Build history of the part. All positions in model axes, mm. Face numbers are marked on the shaded views. A direction names the side the tool comes from. Round coordinates to 2 decimals unless told otherwise and drop trailing zeros. Loops run counter-clockwise (first coordinate to the right, second up) from the corner with the lowest first, then second, coordinate; pieces in that order, holes last. Notation, with made-up numbers: (-35.75, 60.25) - (18.25, 60.25) arc R27 ccw to (18.25, 93.25) - close; hole circle Ø7 at (34, 83.5). An arc over 180 degrees is marked (long way). Put each result on its own line as item: value. Start each with the question number.
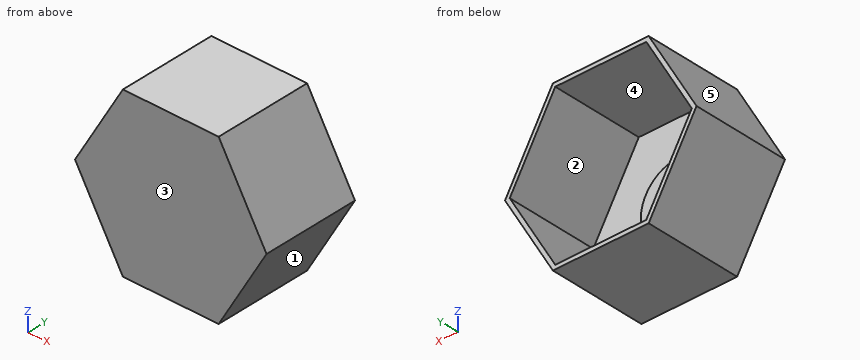
from build123d import *

# Parameters (mm, degrees)
BOSS_EXTRUDE1_DEPTH = 72
CUT_EXTRUDE1_DEPTH  = 68
SKETCH4_R           = 27.5
BOSS_EXTRUDE2_DEPTH = 5


with BuildPart() as part:
    # Sketch2 → Boss-Extrude1 (new body)
    with BuildSketch(Plane(origin=(0, 0, 0), x_dir=(1, 0, 0), z_dir=(0, 1, 0))):
        Polygon((70.436732841, 0), (35.218366421, 61), (-35.218366421, 61), (-70.436732841, 0), (-35.218366421, -61), (35.218366421, -61), align=None)
    extrude(amount=BOSS_EXTRUDE1_DEPTH)

    # Sketch3 → Cut-Extrude1 (cut)
    with BuildSketch(Plane(origin=(0, 72, 0), x_dir=(1, 0, 0), z_dir=(0, 1, 0))):
        Polygon((66.972631226, 0), (33.486315613, 58), (-33.486315613, 58), (-66.972631226, 0), (-33.486315613, -58), (33.486315613, -58), align=None)
    extrude(amount=-CUT_EXTRUDE1_DEPTH, mode=Mode.SUBTRACT)

    # Sketch4 → Boss-Extrude2 (add)
    with BuildSketch(Plane(origin=(0, 4, 0), x_dir=(1, 0, 0), z_dir=(0, 1, 0))):
        with Locations(Location((0, 0, 0), (0, 0, 270))):
            Circle(SKETCH4_R)
    extrude(amount=BOSS_EXTRUDE2_DEPTH)


solid = part.part
Item 1: Drop flat-ended pins along their axis: pin 1 Ø8 at (x, z) = (-44, 5) entering from +Y; pin 2 Ø12 at (y, z) = (8, 19) entering from +X; pin 3 Ø1 at (y, z) = (54, 23) entering from +X. Give the stop position or say it passes through.
Item 2: Slice it at B-B (z = 51). Give the cut face in (x, y).
Item 3: Two-plate mould, pull along X, no slides. Class the marked faces 3, 4 and 5: pulls with the +X half, pulls with the -X half, needs draft (parallel to the pull), parting line crosses it, or undercut.
Item 4: Drill centre lines: probe 1 along Z at (x, y) = (24, 41.5); probe 2 along X at (y, z) = (8.5, 13.5); probe 3 along Y at (x, z) = (2, 47.5). Where is each one in solid material? Low to high. Write a range as [from, to].
Item 5: Which spindle directions (+Z, -Z, +X, -X, +Y, -Y) get a long thin tool onto all of the face, cutting with end or side? Do the marked faces 1 and 2. Say none if no direction does.
Item 6: Slice it at D-D (z = 7). Give the cut face in (x, y).
Item 7: Slice it at A-A (y = 27.5). Give the cut face in (x, z).
Item 8: Slice it at C-C (x = -39.5). Give the cut face in (y, z), plus the area to 3 significant figures.
Computed values:
1. pin 1: stops at y = 4
1. pin 2: stops at x = 62.93
1. pin 3: stops at x = 57.45
2. outline: (-40.99, 0) - (40.99, 0) - (40.99, 72) - (37.53, 72) - (37.53, 4) - (-37.53, 4) - (-37.53, 72) - (-40.99, 72) - close
3. face 3: needs draft
3. face 4: undercut
3. face 5: pulls with the -X half
4. probe 1: z = [-61, -58], [58, 61]
4. probe 2: x = [-62.64, -59.18], [-23.96, 23.96], [59.18, 62.64]
4. probe 3: y = [0, 4]
5. face 1: -Z, +X, +Y, -Y
5. face 2: +Y
6. outline: (-66.4, 0) - (66.4, 0) - (66.4, 72) - (62.93, 72) - (62.93, 4) - (26.59, 4) - (26.59, 9) - (-26.59, 9) - (-26.59, 4) - (-62.93, 4) - (-62.93, 72) - (-66.4, 72) - close
7. outline: (-70.44, 0) - (-35.22, -61) - (35.22, -61) - (70.44, 0) - (35.22, 61) - (-35.22, 61) - close; hole (-66.97, 0) - (-33.49, -58) - (33.49, -58) - (66.97, 0) - (33.49, 58) - (-33.49, 58) - close
8. outline: (0, -53.58) - (72, -53.58) - (72, -47.58) - (4, -47.58) - (4, 47.58) - (72, 47.58) - (72, 53.58) - (0, 53.58) - close
8. area: 1,240 mm^2
